Read the model definition and answer for the solid it produces. Units are mm, in the model's axes. A direction names the side the tool comes from. Coordinates: 2 decimals unless noted, no trailing zeros. Write each loop counter-clockwise with the first axis right and the second up, starting at its lowest first coordinate (ties: lowest second). Pieces come first, ordered by that corner, then holes. Notation, with made-up numbers: (67, -31.5) -> (71, -31.5) arc R22 ccw to (71, -0.5) -> close; hole circle Ø5 at (67.5, 15.5). An arc over 180 degrees is marked (long way). Use CSV: the item, a comma, the result in double quotes.
from build123d import *

# Parameters (mm, degrees)
BOSS_EXTRUDE1_DEPTH = 1.7
SKETCH2_W           = 1.2
SKETCH2_H           = 17.279106444
BOSS_EXTRUDE2_DEPTH = 3.5
CUT_EXTRUDE1_REACH  = 69.63
SKETCH4_W           = 0.999194929
SKETCH4_H           = 30.9
BOSS_EXTRUDE3_DEPTH = 3.5
FILLET1_R           = 2
FILLET2_R           = 0.5
SKETCH5_W           = 5
SKETCH5_H           = 2.5
CUT_EXTRUDE2_DEPTH  = 38.119536635
SKETCH6_W           = 10
SKETCH6_H           = 10
SKETCH6_W_2         = 8
SKETCH6_H_2         = 8
EXTRUDE_THIN1_DEPTH = 2.3
SKETCH8_R           = 1.4
BOSS_EXTRUDE4_DEPTH = 7
SKETCH8_2_R         = 2.4
SKETCH8_2_R_2       = 1.4
EXTRUDE_THIN2_DEPTH = 5.4


with BuildPart() as part:
    # Sketch1 → Boss-Extrude1 (new body)
    with BuildSketch(Plane.XY):
        Polygon((-32.1, 15.6), (30.9, 15.6), (30.9, 14.4), (32.500805071, 14.4), (32.500805071, 15.45), (33.5, 15.45), (33.5, -15.45), (32.500805071, -15.45), (32.500805071, -14.4), (30.9, -14.4), (30.9, -15.6), (-32.1, -15.6), (-32.1, -7.7), (-31.6, -7.7), (-31.6, 7.7), (-32.1, 7.7), align=None)
    extrude(amount=-BOSS_EXTRUDE1_DEPTH)

    # Sketch2 → Boss-Extrude2 (add)
    with BuildSketch(Plane(origin=(0, 0, -1.7), x_dir=(-1, 0, 0), z_dir=(0, 0, -1))):
        with Locations((31.5, -0.060446778)):
            Rectangle(SKETCH2_W, SKETCH2_H)
    extrude(amount=BOSS_EXTRUDE2_DEPTH)

    # Sketch3 → Cut-Extrude1 (cut, up to next)
    with BuildSketch(Plane(origin=(33.5, 0, 0), x_dir=(0, 0, -1), z_dir=(1, 0, 0)), mode=Mode.PRIVATE) as cut_extrude1_sk1:
        Polygon((1.7, 15.45), (0, 15.45), (1.7, 14.883333333), align=None)
    cut_extrude1_tool1 = extrude(cut_extrude1_sk1.sketch, amount=-CUT_EXTRUDE1_REACH, mode=Mode.PRIVATE) & part.part
    cut_extrude1 = cut_extrude1_tool1.solids().sort_by_distance((33.5, 15.261111, -1.133333))[0]
    add(cut_extrude1, mode=Mode.SUBTRACT)

    # Mirror1: Cut-Extrude1 across plane
    add(cut_extrude1.mirror(Plane.ZX), mode=Mode.SUBTRACT)

    # Sketch4 → Boss-Extrude3 (add)
    with BuildSketch(Plane(origin=(0, 0, -1.7), x_dir=(-1, 0, 0), z_dir=(0, 0, -1))):
        with Locations((-33.000402536, 0)):
            Rectangle(SKETCH4_W, SKETCH4_H)
    extrude(amount=BOSS_EXTRUDE3_DEPTH)

    # Fillet1
    fillet1_edges = [part.edges().sort_by_distance(p)[0] for p in [
        (-32.1, -15.6, -0.85),
        (-32.1, 15.6, -0.85),
    ]]
    fillet(fillet1_edges, radius=FILLET1_R)

    # Fillet2
    fillet2_edges = [part.edges().sort_by_distance(p)[0] for p in [
        (33.5, 0, 0),
    ]]
    fillet(fillet2_edges, radius=FILLET2_R)

    # Sketch5 → Cut-Extrude2 (cut, through all)
    with BuildSketch(Plane(origin=(0, 0, -1.7), x_dir=(-1, 0, 0), z_dir=(0, 0, -1))):
        with Locations((-16, -6.35)):
            Rectangle(SKETCH5_W, SKETCH5_H)
        with Locations((-16, -2.45)):
            Rectangle(SKETCH5_W, SKETCH5_H)
        with Locations((-16, 1.45)):
            Rectangle(SKETCH5_W, SKETCH5_H)
        with Locations((-23.9, 5.35)):
            Rectangle(SKETCH5_W, SKETCH5_H)
    extrude(amount=-CUT_EXTRUDE2_DEPTH, mode=Mode.SUBTRACT)

    # Sketch6 → Extrude-Thin1 (add)
    with BuildSketch(Plane(origin=(0, 0, -1.7), x_dir=(-1, 0, 0), z_dir=(0, 0, -1))):
        with Locations((12.508033049, -0.060446778)):
            Rectangle(SKETCH6_W, SKETCH6_H)
        with Locations((12.508033049, -0.060446778)):
            Rectangle(SKETCH6_W_2, SKETCH6_H_2, mode=Mode.SUBTRACT)
    extrude(amount=EXTRUDE_THIN1_DEPTH)

    # Sketch8 → Boss-Extrude4 (add)
    with BuildSketch(Plane(origin=(0, 0, -1.7), x_dir=(-1, 0, 0), z_dir=(0, 0, -1))):
        with Locations(Location((-22.549962349, -9.941736634, 0), (0, 0, 270))):
            Circle(SKETCH8_R)
        with Locations(Location((-17.469962349, 7.838263366, 0), (0, 0, 270))):
            Circle(SKETCH8_R)
    extrude(amount=BOSS_EXTRUDE4_DEPTH)

    # Sketch8<2> → Extrude-Thin2 (add)
    # profile 1 of 2: a face of its own
    with BuildSketch(Plane(origin=(0, 0, -1.7), x_dir=(-1, 0, 0), z_dir=(0, 0, -1))):
        with Locations((-22.549962349, -9.941736634)):
            Circle(SKETCH8_2_R)
        with Locations((-22.549962349, -9.941736634)):
            Circle(SKETCH8_2_R_2, mode=Mode.SUBTRACT)
    # profile 2 of 2: a face of its own
    with BuildSketch(Plane(origin=(0, 0, -1.7), x_dir=(-1, 0, 0), z_dir=(0, 0, -1))):
        with Locations((-17.469962349, 7.838263366)):
            Circle(SKETCH8_2_R)
        with Locations((-17.469962349, 7.838263366)):
            Circle(SKETCH8_2_R_2, mode=Mode.SUBTRACT)
    extrude(amount=EXTRUDE_THIN2_DEPTH)


solid = part.part
1. A cutting plane is placed at A-A (y = -6). Give the vertices of the cut face in (x, z), and give its area (3 significant figures).
Solutions:
outline,"(-32.1, -5.2) -> (-30.9, -5.2) -> (-30.9, -1.7) -> (13.5, -1.7) -> (13.5, 0) -> (-31.6, 0) -> (-31.6, -1.7) -> (-32.1, -1.7) -> close; (18.5, -1.7) -> (32.5, -1.7) -> (32.5, -5.2) -> (33.5, -5.2) -> (33.5, -0.5) arc R0.5 ccw to (33, 0) -> (18.5, 0) -> close"
area,"110 mm^2"
2. For a pull along Y with two mould halves and no side action, classify faces 6 (the flat face through (-31.5, 8.579, -3.4)), 7 (the cylindrical face through (24.948, -9.836, -4.362)), 8 (the flat face through (18.5, -2, -1)), 9 (the flat face through (-32.1, 0, -3)) as pulls with the +Y half, pulls with the -Y half, needs draft (parallel to the pull), parting line crosses it, or undercut.
Solutions:
face 6,"pulls with the +Y half"
face 7,"parting line crosses it"
face 8,"undercut"
face 9,"needs draft"
3. Each of these flat-tipped pins is pushed along its axis until it touches: pin 1 Ø4 at (x, y) = (-12.5, -1) entering from -Z; pin 2 Ø0.5 at (x, y) = (33, -7) entering from -Z; pin 3 Ø8 at (x, y) = (-15, 2) entering from -Z. Where does it stop, or does it pass through?
Solutions:
pin 1,"stops at z = -1.7"
pin 2,"stops at z = -5.2"
pin 3,"stops at z = -4"
4. A cutting plane is placed at C-C (y = 1). Give the vertices of the cut face in (x, z), and give its area (3 significant figures).
Solutions:
outline,"(-32.1, -5.2) -> (-30.9, -5.2) -> (-30.9, -1.7) -> (-17.51, -1.7) -> (-17.51, -4) -> (-16.51, -4) -> (-16.51, -1.7) -> (-8.51, -1.7) -> (-8.51, -4) -> (-7.51, -4) -> (-7.51, -1.7) -> (13.5, -1.7) -> (13.5, 0) -> (-31.6, 0) -> (-31.6, -1.7) -> (-32.1, -1.7) -> close; (18.5, -1.7) -> (32.5, -1.7) -> (32.5, -5.2) -> (33.5, -5.2) -> (33.5, -0.5) arc R0.5 ccw to (33, 0) -> (18.5, 0) -> close"
area,"114 mm^2"
5. A cutting plane is placed at B-B (y = 11). Give the vertices of the cut face in (x, z).
Solutions:
outline,"(-32.1, -1.7) -> (32.5, -1.7) -> (32.5, -5.2) -> (33.5, -5.2) -> (33.5, -0.5) arc R0.5 ccw to (33, 0) -> (-32.1, 0) -> close"
6. A cutting plane is placed at D-D (x = -5). Give the vertices of the cut face in (y, z), and give its area (3 significant figures).
Solutions:
outline,"(-15.6, -1.7) -> (15.6, -1.7) -> (15.6, 0) -> (-15.6, 0) -> close"
area,"53.0 mm^2"
7. Find the intervals of material crossed by line 1 along X through (y, z) = (-7, -2.75); line 2 along Y through (x, z) = (16.5, -0.75); line 3 along X through (y, z) = (-4, -3.75), in increasing order.
Solutions:
line 1,"x = -32.1 to -30.9, 32.5 to 33.5"
line 2,"y = -15.6 to -7.6, -5.1 to -3.7, -1.2 to 0.2, 2.7 to 15.6"
line 3,"x = -32.1 to -30.9, -17.51 to -16.51, -8.51 to -7.51, 32.5 to 33.5"
8. A tool of negligible diameter and unlimited length cuts with its end or side. For faces 1 (the flat face through (32, 14.4, -1)), 2 (the flat face through (-7.508, 0, -3)), 3 (the flat face through (-16.508, 0, -3)), 4 (the flat face through (-31.6, 0, -1)), 5 (the flat face through (16, -5.1, -1)), from which of +Z, -Z, +X, -X, +Y, -Y can it reach the whole face along a straight path? Write none if from no direction.
Solutions:
face 1,"+Z, -Z, +Y"
face 2,"-Z, +Y, -Y"
face 3,"-Z"
face 4,"+Z, -X"
face 5,"+Z, -Z"
